from build123d import *

# Parameters (mm, degrees)
BOSS_EXTRUDE1_DEPTH     = 10.325
CUT_EXTRUDE4_DEPTH      = 35.751582698
CUT_EXTRUDE4_DEPTH_BACK = 35.751582698
SKETCH4_W               = 0.25
SKETCH4_H               = 3
CUT_EXTRUDE5_DEPTH      = 35.751582698
CUT_EXTRUDE5_DEPTH_BACK = 35.751582698
SKETCH5_R               = 1
FILLET5_R               = 2
BOSS_EXTRUDE2_START     = 2
BOSS_EXTRUDE2_DEPTH     = 2
SKETCH7_W               = 10.16
SKETCH7_H               = 3.425
CUT_EXTRUDE6_DEPTH      = 37.305250358


with BuildPart() as part:
    # Sketch1 → Boss-Extrude1 (new, symmetric)
    with BuildSketch(Plane(origin=(0, 0, 0), x_dir=(1, 0, 0), z_dir=(0, 1, 0))):
        Polygon((-15, -12.5), (15, -12.5), (25, -12.5), (15, 2.5), (14.20625, 2.5), (14.20625, 5.5), (9.20625, 5.5), (9.20625, 12.5), (-9.20625, 12.5), (-9.20625, 5.5), (-14.20625, 5.5), (-14.20625, 2.5), (-15, 2.5), (-25, -12.5), align=None)
    extrude(amount=BOSS_EXTRUDE1_DEPTH, both=True)

    # Sketch4 → Cut-Extrude4 (cut, two sides: drawn at the far end of the back side and taken through both)
    with BuildSketch(Plane(origin=(0, 10.325, 0), x_dir=(1, 0, 0), z_dir=(0, 1, 0)).offset(-CUT_EXTRUDE4_DEPTH_BACK)):
        with Locations((14.08125, 4)):
            Rectangle(SKETCH4_W, SKETCH4_H)
        with Locations((-14.08125, 4)):
            Rectangle(SKETCH4_W, SKETCH4_H)
    extrude(amount=CUT_EXTRUDE4_DEPTH + CUT_EXTRUDE4_DEPTH_BACK, mode=Mode.SUBTRACT)

    # Sketch5 → Cut-Extrude5 (cut, two sides: drawn at the far end of the back side and taken through both)
    with BuildSketch(Plane(origin=(0, 10.325, 0), x_dir=(1, 0, 0), z_dir=(0, 1, 0)).offset(-CUT_EXTRUDE5_DEPTH_BACK)):
        with Locations((-14.663356781, 3.207106781)):
            Circle(SKETCH5_R)
        with Locations((14.663356781, 3.207106781)):
            Circle(SKETCH5_R)
    extrude(amount=CUT_EXTRUDE5_DEPTH + CUT_EXTRUDE5_DEPTH_BACK, mode=Mode.SUBTRACT)

    # Fillet5
    fillet5_edges = [part.edges().sort_by_distance(p)[0] for p in [
        (-25, 0, 12.5),
        (-9.20625, 0, -5.5),
        (9.20625, 0, -5.5),
        (25, 0, 12.5),
    ]]
    fillet(fillet5_edges, radius=FILLET5_R)

    # Sketch6 → Boss-Extrude2 (add)
    with BuildSketch(Plane(origin=(0, 10.325, 0), x_dir=(1, 0, 0), z_dir=(0, 1, 0)).offset(BOSS_EXTRUDE2_START)):
        with BuildLine():
            Line((-14.053996179, 4), (-7.5, 4))
            Line((-7.5, 4), (-7.5, 1))
            Line((-7.5, 1), (-16, 1))
            Line((-16, 1), (-15.121262614, 2.318106079))
            ThreePointArc((-15.121262614, 2.318106079), (-13.819007075, 2.671314309), (-14.053996179, 4))
        make_face()
        with BuildLine():
            Line((16, 1), (15.121262614, 2.318106079))
            ThreePointArc((15.121262614, 2.318106079), (13.819007075, 2.671314309), (14.053996179, 4))
            Line((14.053996179, 4), (7.5, 4))
            Line((7.5, 4), (7.5, 1))
            Line((7.5, 1), (16, 1))
        make_face()
    extrude(amount=-BOSS_EXTRUDE2_DEPTH)

    # Sketch7 → Cut-Extrude6 (cut, through all)
    with BuildSketch(Plane.XY.offset(12.5)):
        with Locations((0, 8.6125)):
            Rectangle(SKETCH7_W, SKETCH7_H)
    extrude(amount=-CUT_EXTRUDE6_DEPTH, mode=Mode.SUBTRACT)


solid = part.part
For this review, take the finished solid that the model builds, in its own axes (mm). A direction names the side the tool comes from. Round coordinates to 2 decimals unless told otherwise and drop trailing zeros. Write each loop counter-clockwise with the first axis right and the second up, starting at its lowest first coordinate (ties: lowest second). Pieces come first, ordered by that corner, then holes. Notation, with made-up numbers: (-37, 3) - (-17, 3) arc R26 ccw to (-17, 20) - close; hole circle Ø9 at (-8.5, 14). An arc over 180 degrees is marked (long way). Write item = value, one per line. Start each with the question number.
1. Consider section B-B on z = -10. State the section outline as (x, y) points (3 decimals), plus the area to 3 significant figures.
2. For faces 1 (the face through (-13, 0, -5.5)), 2 (the face through (7.5, 11, -3)), 3 (the face through (-12, 11, -1)), 4 (the face through (-11, 12.325, -3)), 5 (the face through (11, 11, -4)), list the 3-axis set-ups (+Z, -Z, +X, -X, +Y, -Y) from which the entire face can be reached by the end or side of a thin tool; tool diameter is ignored.
3. For pin 1 Ø3 at (x, z) = (1.5, 6) entering from +Y; pin 2 Ø6 at (y, z) = (-7.5, -6.5) entering from -X; pin 3 Ø8 at (y, z) = (7, -3.5) entering from -X, all flat-tipped, find the tip position at first contact; note any pin that passes through.
4. Consider section A-A on y = 9.5. State the section outline as (x, z) points.
5. Wall thickness on L1, parallel to X at y = -2, z = -5; L2, parallel to X at y = -7, z = -9.25; L3, parallel to X at y = 7.5, z = 10.25: over which ranges is each line inside the solid? List them lowest first.
6. Consider section D-D on x = 6.5. State the section outline as (y, z) points (3 decimals), plus the area to 3 significant figures.
7. Consider section C-C on y = -4.5. State the section outline as (x, z) points, plus the area to 3 significant figures.
8. Draft analysis for pull direction X (two halves, no side actions). For faces 6 (the face through (-5.08, 9, 0)), 7 (the face through (23.04, -0.14, 11.42)), 8 (the face through (11, 12.325, -3)), state which applies: released by +X, released by -X, zero draft, split by the parting line, or undercut.
Evaluation:
q1.outline = (-9.206, -10.325) - (9.206, -10.325) - (9.206, 10.325) - (5.08, 10.325) - (5.08, 6.9) - (-5.08, 6.9) - (-5.08, 10.325) - (-9.206, 10.325) - close
q1.area = 345 mm2
q2.face_1 = -Z, -X, +Y, -Y
q2.face_2 = +Z, -Z, +Y
q2.face_3 = +Z, +X, -X, +Y
q2.face_4 = +Z, -Z, +X, -X, +Y
q2.face_5 = -Z, +X, -X, +Y
q3.pin_1 = 6.9
q3.pin_2 = -13.96
q3.pin_3 = -17
q4.outline = (-22.93, 9.39) - (-15.12, -2.32) arc R1 cw to (-13.96, -3.91) - (-13.96, -5.5) - (-11.21, -5.5) arc R2 cw to (-9.21, -7.5) - (-9.21, -12.5) - (-5.08, -12.5) - (-5.08, 12.5) - (-21.26, 12.5) arc R2 ccw to start; (5.08, -12.5) - (9.21, -12.5) - (9.21, -7.5) arc R2 cw to (11.21, -5.5) - (13.96, -5.5) - (13.96, -3.91) arc R1 cw to (15.12, -2.32) - (22.93, 9.39) arc R2 ccw to (21.26, 12.5) - (5.08, 12.5) - close
q5.L1 = -13.96 to 13.96
q5.L2 = -9.21 to 9.21
q5.L3 = -23.25 to -5.08, 5.08 to 23.25
q6.outline = (-10.325, -12.5) - (10.325, -12.5) - (10.325, 12.5) - (-10.325, 12.5) - close
q6.area = 516 mm2
q7.outline = (-22.93, 9.39) - (-15.12, -2.32) arc R1 cw to (-13.96, -3.91) - (-13.96, -5.5) - (-11.21, -5.5) arc R2 cw to (-9.21, -7.5) - (-9.21, -12.5) - (9.21, -12.5) - (9.21, -7.5) arc R2 cw to (11.21, -5.5) - (13.96, -5.5) - (13.96, -3.91) arc R1 cw to (15.12, -2.32) - (22.93, 9.39) arc R2 ccw to (21.26, 12.5) - (-21.26, 12.5) arc R2 ccw to start
q7.area = 807 mm2
q8.face_6 = undercut
q8.face_7 = released by +X
q8.face_8 = zero draft
